```python
from build123d import *

# Parameters (mm, degrees)
SKETCH_1_W          = 118.3
SKETCH_1_H          = 44.2
EXTRUDE_1_DEPTH     = 2.8
SKETCH_2_W          = 2.8
SKETCH_2_H          = 44.2
CUT_EXTRUDE_1_DEPTH = 1
CUT_EXTRUDE_2_DEPTH = 122.622082534


with BuildPart() as part:
    # 草图1 → 凸台-拉伸1 (new body)
    with BuildSketch(Plane(origin=(0, 0, 0), x_dir=(1, 0, 0), z_dir=(0, 1, 0))):
        with Locations((13.975775656, 5.992720764)):
            Rectangle(SKETCH_1_W, SKETCH_1_H)
    extrude(amount=EXTRUDE_1_DEPTH)

    # 草图2 → 切除-拉伸1 (cut)
    with BuildSketch(Plane(origin=(0, 2.8, 0), x_dir=(1, 0, 0), z_dir=(0, 1, 0))):
        with Locations((-43.774224344, 5.992720764)):
            Rectangle(SKETCH_2_W, SKETCH_2_H)
        with Locations((71.725775656, 5.992720764)):
            Rectangle(SKETCH_2_W, SKETCH_2_H)
    extrude(amount=-CUT_EXTRUDE_1_DEPTH, mode=Mode.SUBTRACT)

    # 草图3 → 切除-拉伸2 (cut, through all)
    with BuildSketch(Plane.ZY.offset(45.174224344)):
        Polygon((-28.092720764, 0), (-28.092720764, 2.8), (-25.292720764, 2.8), align=None)
        Polygon((16.107279236, 0), (16.107279236, 2.8), (13.307279236, 2.8), align=None)
    extrude(amount=-CUT_EXTRUDE_2_DEPTH, mode=Mode.SUBTRACT)


solid = part.part
```
Here's how the part is built. I have some questions about the finished solid (model axes, mm). A direction names the side the tool comes from. Give positions to 0.01 mm unless a question says otherwise; leave off trailing zeros. Order: outer loops, then holes, each group sorted by start corner. A loop starts at its lowest first (then second) coordinate and runs counter-clockwise, first axis right, second up. Notation, with made-up numbers: M 68,-8 L 79,-8 A23 ccw 79,28 Z; hole C -28,-36.75 d9. An arc over 180 degrees is marked long. Use a Markdown table: item, result. Add a question column.
1. I need wall thicknesses on probe 1 along X at (y, z) = (2.5, 8); probe 2 along Z at (x, y) = (39.5, 0.7); probe 3 along Z at (x, y) = (35, 0.55). Which ranges of each line are inside material? Lowest first, please. Write a range as from..to.
2. For pin 1 Ø0.8 at (x, z) = (71.5, -13.5) entering from +Y; pin 2 Ø0.8 at (y, z) = (2.5, -9) entering from +X, each with a flat end and sliding along its axis, tell me the tip position at first contact or that it passes through.
3. Suppose I cut it at A-A (z = -8). List the corners of the cut face in (x, y) for me, and give its area (3 significant figures).
4. Suppose I cut it at C-C (x = -13). List the corners of the cut face in (y, z) for me.
5. Suppose I cut it at B-B (y = 2.35). List the corners of the cut face in (x, z) for me.
6. On a 3-axis mill with a long thin cutter (end or side, diameter ignored), from which of +Z, -Z, +X, -X, +Y, -Y can I reach the whole of each face in a straight line? I mean faces 1 (the flat face through (13.15, 1.42, -26.67)), 2 (the flat face through (72, 1.8, -6)), 3 (the flat face through (-44, 1.8, -6)). Say none if no direction works.
Results list:
| question | item | result |
|---|---|---|
| 1 | probe 1 | x = -42.37..70.33 |
| 1 | probe 2 | z = -27.39..15.41 |
| 1 | probe 3 | z = -27.54..15.56 |
| 2 | pin 1 | stops at y = 1.8 |
| 2 | pin 2 | stops at x = 70.33 |
| 3 | outline | M -45.17,0 L 73.13,0 L 73.13,1.8 L 70.33,1.8 L 70.33,2.8 L -42.37,2.8 L -42.37,1.8 L -45.17,1.8 Z |
| 3 | area | 326 mm² |
| 4 | outline | M 0,-28.09 L 2.8,-25.29 L 2.8,13.31 L 0,16.11 Z |
| 5 | outline | M -42.37,-25.74 L 70.33,-25.74 L 70.33,13.76 L -42.37,13.76 Z |
| 6 | face 1 | -Z, +X, -X, +Y |
| 6 | face 2 | +Z, -Z, +X, +Y |
| 6 | face 3 | +Z, -Z, -X, +Y |
